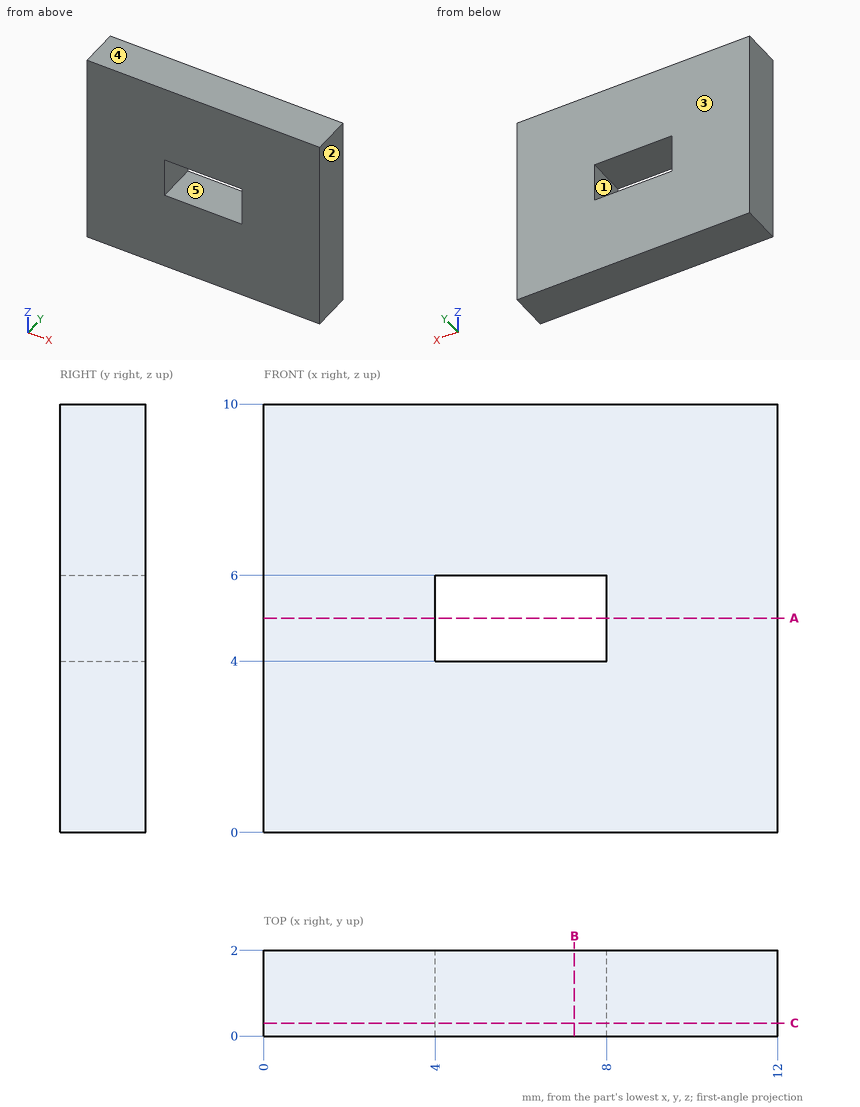
Could you check a few things on this drawing? It's one solid part, dimensions in mm from its lowest x, y, z. A direction names the side the tool comes from. Coordinates: 2 decimals unless noted, no trailing zeros. Order: outer loops, then holes, each group sorted by start corner. A loop starts at its lowest first (then second) coordinate and runs counter-clockwise, first axis right, second up.
1) We'd pull the mould along X, two halves only. Please class the marked faces 1, 2 and 3: +X half, -X half, draft (parallel to the pull), parting line (faces both ways), or undercut.
2) I need wall thicknesses on line 1 (Z direction, x = 6.5, y = 1.45); line 2 (X direction, y = 1.1, z = 5.75). Which ranges of each line are inside material? Lowest first, please.
3) Imagine slicing it at B-B on x = 7.25. List the corners of the cut face in (y, z) for me, and give its area (3 significant figures).
4) Which directions (+Z, -Z, +X, -X, +Y, -Y) give clear straight access to the entire face, cutting with the end or side of a thin tool? Please do the marked faces 4 and 5.
5) Imagine slicing it at A-A on z = 5. List the corners of the cut face in (x, y) for me, and give its area (3 significant figures).
6) Imagine slicing it at C-C on y = 0.3. List the corners of the cut face in (x, z) for me.
Response values:
1. face 1: undercut
1. face 2: +X half
1. face 3: draft
2. line 1: z = 0 to 4, 6 to 10
2. line 2: x = 0 to 4, 8 to 12
3. outline: (0, 0) - (2, 0) - (2, 4) - (0, 4) - close; (0, 6) - (2, 6) - (2, 10) - (0, 10) - close
3. area: 16.0 mm2
4. face 4: +Z, +X, -X, +Y, -Y
4. face 5: +Y, -Y
5. outline: (0, 0) - (4, 0) - (4, 2) - (0, 2) - close; (8, 0) - (12, 0) - (12, 2) - (8, 2) - close
5. area: 16.0 mm2
6. outline: (0, 0) - (12, 0) - (12, 10) - (0, 10) - close; hole (4, 4) - (8, 4) - (8, 6) - (4, 6) - close
